Build history of the part. All positions in model axes, mm. A direction names the side the tool comes from. Round coordinates to 2 decimals unless told otherwise and drop trailing zeros. Write each loop counter-clockwise with the first axis right and the second up, starting at its lowest first coordinate (ties: lowest second). Pieces come first, ordered by that corner, then holes. Notation, with made-up numbers: (-26, 39) -> (-8, 39) arc R14 cw to (-8, 57) -> close; hole circle Ø9 at (5.25, -27.5). An arc over 180 degrees is marked (long way). Answer in a Markdown table with one row per item. Add a question column.
from build123d import *

# Parameters (mm, degrees)
SKETCH2_R           = 2.75
SKETCH2_W           = 60
SKETCH2_H           = 20
BOSS_EXTRUDE1_DEPTH = 5


with BuildPart() as part:
    # Sketch2 → Boss-Extrude1 (new body)
    with BuildSketch(Plane(origin=(0, 0, 0), x_dir=(1, 0, 0), z_dir=(0, 1, 0))):
        Polygon((-60, 30), (0, 30), (0, 130), (-20, 130), (-60, 130), (-86.701035329, 73.505676753), align=None)
        with Locations((-60, 85)):
            Circle(SKETCH2_R, mode=Mode.SUBTRACT)
        with Locations((-20, 105)):
            Circle(SKETCH2_R, mode=Mode.SUBTRACT)
        Polygon((0, 130), (0, 30), (60, 30), (86.701035329, 73.505676753), (60, 130), (20, 130), align=None)
        with Locations((60, 85)):
            Circle(SKETCH2_R, mode=Mode.SUBTRACT)
        with Locations((20, 105)):
            Circle(SKETCH2_R, mode=Mode.SUBTRACT)
        with Locations((-30, 20)):
            Rectangle(SKETCH2_W, SKETCH2_H)
        with Locations((30, 20)):
            Rectangle(SKETCH2_W, SKETCH2_H)
    extrude(amount=BOSS_EXTRUDE1_DEPTH)


solid = part.part
(1) Probe line 1 along Z through (x, y) = (-20, 2.3); line 2 along X through (y, z) = (3.3, -85); line 3 along X through (y, z) = (1.75, -105). List the from-to ranges inside material, lowest first.
(2) Drop flat-ended pins along their axis: P1, Ø7, axis at x = -60, z = -85, coming from the -Y side; P2, Ø1, axis at y = 3.5, z = -69.5, coming from the +X side. Give the stop position or say it passes through.
(3) Saw through at A-A (y = 2.9). List the corners of the cut face in (x, z), plus the area to 3 significant figures.
(4) Mould opens along Z. For faces 4 (the face through (73.537, 2.465, -101.357)), 5 (the face through (19.404, 2.465, -102.315)), 6 (the face through (-20.596, 2.465, -102.315)), 7 (the face through (73.164, 2.465, -51.448)) say: pulls with the +Z half, pulls with the -Z half, needs draft (parallel to the pull), parting line crosses it, or undercut.
(5) Saw through at C-C (z = -85). List the corners of the cut face in (x, y), plus the area to 3 significant figures.
(6) Saw through at B-B (x = 20). List the corners of the cut face in (y, z), plus the area to 4 significant figures.
(7) Which spindle directions (+Z, -Z, +X, -X, +Y, -Y) get a long thin tool onto all of the face, cutting with end or side? Do faces 1 (the face through (-73.164, 2.465, -102.148)), 2 (the face through (60, 2, -20)), 3 (the face through (-60, 2, -20)). Say none if no direction does.
(8) Saw through at D-D (z = -118.5). List the corners of the cut face in (x, y), plus the area to 3 significant figures.
Answer sheet:
| question | item | result |
|---|---|---|
| 1 | line 1 | z = -130 to -107.75, -102.25 to -10 |
| 1 | line 2 | x = -81.27 to -62.75, -57.25 to 57.25, 62.75 to 81.27 |
| 1 | line 3 | x = -71.82 to -22.75, -17.25 to 17.25, 22.75 to 71.82 |
| 2 | P1 | stops at y = 0 |
| 2 | P2 | stops at x = 84.55 |
| 3 | outline | (-86.7, -73.51) -> (-60, -130) -> (60, -130) -> (86.7, -73.51) -> (60, -30) -> (60, -10) -> (-60, -10) -> (-60, -30) -> close; hole circle Ø5.5 at (-60, -85); hole circle Ø5.5 at (-20, -105); hole circle Ø5.5 at (20, -105); hole circle Ø5.5 at (60, -85) |
| 3 | area | 17,000 mm² |
| 4 | face 4 | pulls with the -Z half |
| 4 | face 5 | undercut |
| 4 | face 6 | undercut |
| 4 | face 7 | pulls with the +Z half |
| 5 | outline | (-81.27, 0) -> (-62.75, 0) -> (-62.75, 5) -> (-81.27, 5) -> close; (-57.25, 0) -> (57.25, 0) -> (57.25, 5) -> (-57.25, 5) -> close; (62.75, 0) -> (81.27, 0) -> (81.27, 5) -> (62.75, 5) -> close |
| 5 | area | 758 mm² |
| 6 | outline | (0, -130) -> (5, -130) -> (5, -107.75) -> (0, -107.75) -> close; (0, -102.25) -> (5, -102.25) -> (5, -10) -> (0, -10) -> close |
| 6 | area | 572.5 mm² |
| 7 | face 1 | -Z, -X, +Y, -Y |
| 7 | face 2 | +Z, +X, +Y, -Y |
| 7 | face 3 | +Z, -X, +Y, -Y |
| 8 | outline | (-65.44, 0) -> (65.44, 0) -> (65.44, 5) -> (-65.44, 5) -> close |
| 8 | area | 654 mm² |
